from build123d import *

# Parameters (mm, degrees)
SKETCH_1_W          = 250
SKETCH_1_H          = 160
EXTRUDE_1_DEPTH     = 6
SKETCH_2_R          = 1.5
CUT_EXTRUDE_1_DEPTH = 6
SKETCH_3_R          = 1.5
SKETCH_3_R_2        = 4
SKETCH_3_W          = 13
SKETCH_3_H          = 20
CUT_EXTRUDE_2_DEPTH = 6
SKETCH_4_W          = 15
SKETCH_4_H          = 30
CUT_EXTRUDE_3_DEPTH = 6


with BuildPart() as part:
    # Эскиз1 → Бобышка-Вытянуть1 (new body)
    with BuildSketch(Plane(origin=(0, 0, 0), x_dir=(1, 0, 0), z_dir=(0, 1, 0))):
        with Locations((55.297029703, 1.056105611)):
            Rectangle(SKETCH_1_W, SKETCH_1_H)
    extrude(amount=EXTRUDE_1_DEPTH)

    # Эскиз2 → Вырез-Вытянуть1 (cut)
    with BuildSketch(Plane(origin=(0, 6, 0), x_dir=(1, 0, 0), z_dir=(0, 1, 0))):
        with Locations(Location((-39.702970297, 71.056105611, 0), (0, 0, 270))):
            Circle(SKETCH_2_R)
        with Locations(Location((-59.702970297, 51.056105611, 0), (0, 0, 90))):
            Circle(SKETCH_2_R)
        with Locations(Location((150.297029703, 71.056105611, 0), (0, 0, 90))):
            Circle(SKETCH_2_R)
        with Locations(Location((170.297029703, 51.056105611, 0), (0, 0, 270))):
            Circle(SKETCH_2_R)
        with Locations(Location((170.297029703, -48.943894389, 0), (0, 0, 90))):
            Circle(SKETCH_2_R)
        with Locations(Location((150.297029703, -68.943894389, 0), (0, 0, 270))):
            Circle(SKETCH_2_R)
        with Locations(Location((-59.702970297, -48.943894389, 0), (0, 0, 270))):
            Circle(SKETCH_2_R)
        with Locations(Location((-39.702970297, -68.943894389, 0), (0, 0, 90))):
            Circle(SKETCH_2_R)
        with Locations(Location((35.297029703, 1.056105611, 0), (0, 0, 270))):
            Circle(SKETCH_2_R)
        with Locations(Location((55.297029703, 21.056105611, 0), (0, 0, 90))):
            Circle(SKETCH_2_R)
        with Locations(Location((55.297029703, -18.943894389, 0), (0, 0, 90))):
            Circle(SKETCH_2_R)
        with Locations(Location((75.297029703, 1.056105611, 0), (0, 0, 270))):
            Circle(SKETCH_2_R)
    extrude(amount=-CUT_EXTRUDE_1_DEPTH, mode=Mode.SUBTRACT)

    # Эскиз3 → Вырез-Вытянуть2 (cut)
    with BuildSketch(Plane(origin=(0, 6, 0), x_dir=(1, 0, 0), z_dir=(0, 1, 0))):
        with Locations(Location((140.297029703, 31.056105611, 0), (0, 0, 270))):
            Circle(SKETCH_3_R)
        with Locations(Location((120.297029703, 31.056105611, 0), (0, 0, 270))):
            Circle(SKETCH_3_R)
        with Locations(Location((130.297029703, 31.056105611, 0), (0, 0, 270))):
            Circle(SKETCH_3_R_2)
        with Locations((143.797029703, 1.056105611)):
            Rectangle(SKETCH_3_W, SKETCH_3_H)
    extrude(amount=-CUT_EXTRUDE_2_DEPTH, mode=Mode.SUBTRACT)

    # Эскиз4 → Вырез-Вытянуть3 (cut)
    with BuildSketch(Plane(origin=(0, 6, 0), x_dir=(1, 0, 0), z_dir=(0, 1, 0))):
        with Locations((-12.202970297, 1.056105611)):
            Rectangle(SKETCH_4_W, SKETCH_4_H)
    extrude(amount=-CUT_EXTRUDE_3_DEPTH, mode=Mode.SUBTRACT)


solid = part.part
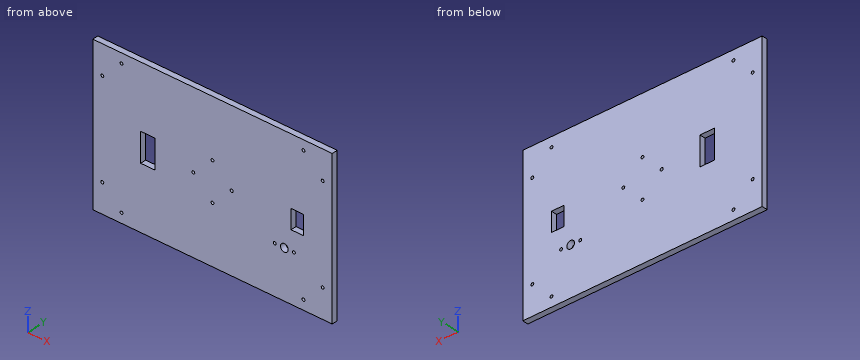
Build history of the part. All positions in model axes, mm. Give positions to 0.01 mm unless a question says otherwise; leave off trailing zeros. Use one line per item in the form item = value.
1) Saw through at A-A (y = 2.5). State how many separate pieces and enclosed holes the cut face has, plus the area to 3 significant figures.
Calculated:
separate_pieces = 1
enclosed_holes = 17
area = 39,100 mm2
2) Probe probe 1 along Z at (x, y) = (150.5, 1.2); probe 2 along Z at (x, y) = (55.5, 1); probe 3 along X at (y, z) = (4.5, -5). List the from-to ranges inside material, lowest first.
Calculated:
probe_1 = -81.06 to -72.54, -69.57 to 67.46, 70.43 to 78.94
probe_2 = -81.06 to -22.54, -19.57 to 17.46, 20.43 to 78.94
probe_3 = -69.7 to -19.7, -4.7 to 137.3, 150.3 to 180.3
3) Drop flat-ended pins along their axis: pin 1 (8 mm diameter, centred on x = -36, z = -57.5, fed in from -Y); pin 2 (1.8 mm diameter, centred on x = 150.3, z = 68.94, fed in from +Y). Give the stop position or say it passes through.
Calculated:
pin_1 = 0
pin_2 = through
